Source: CAD feature listing. Evaluate the final solid. Frame: model axes, mm. Coordinates: 2 decimals unless noted, no trailing zeros. Loops run counter-clockwise (first coordinate to the right, second up) from the corner with the lowest first, then second, coordinate; pieces in that order, holes last. Notation, with made-up numbers: M 17.25,22 L 57.25,22 A28 ccw 57.25,52 Z; hole C 47,57.25 d11. An arc over 180 degrees is marked long. One line per question, with ' | ' between items. Start each with the question number.
1. Mould query, pull axis Z, two halves, no side actions, for faces 1 (the flat face through (-11.5, 1, -10)), 2 (the cylindrical face through (-1.39, 1.48, -16.01)), 3 (the flat face through (-6, 1, 0)), 4 (the cylindrical face through (-1.3, 1.5, -4.1)). Classes: pulls with the +Z half, pulls with the -Z half, needs draft (parallel to the pull), parting line crosses it, or undercut.
2. Section query C-C, the plane y = 1.65. Output: boundary loops of the cut face in (x, z).
3. Ray query, probe 1 along Z at (x, y) = (-9, 1.5); probe 2 along X at (y, z) = (1.4, -6.25); probe 3 along Z at (x, y) = (-1.25, 0.85). Return the intervals inside material, ascending.
4. Section query B-B, the plane x = -9. Output: boundary loops of the cut face in (y, z), and give its area (3 significant figures).
5. Section query A-A, the plane z = -5. Output: boundary loops of the cut face in (x, y), and give its area (3 significant figures).
Autodesk Inventor part; units mm, degrees
ref_plane "YZ Plane" through (0, 0, 0) normal (1, 0, 0) x (0, 1, 0)
ref_plane "XZ Plane" through (0, 0, 0) normal (0, 1, 0) x (-1, 0, 0)
ref_plane "XY Plane" through (0, 0, 0) normal (0, 0, 1) x (1, 0, 0)
sketch "Esquisse1" plane through (0, 0, 0) normal (0, 1, 0) x (-1, 0, 0)
  line L0 (0, 0) -> (11.5, 0)
  line L1 (11.5, 0) -> (11.5, -20)
  line L2 (11.5, -20) -> (0, -20)
  line L3 (0, -20) -> (0, 0)
  line L4 (9, 0) -> (9, -20) construction
  line L5 (5.75, 0) -> (5.75, -20) construction
  line L6 (11.5, -10) -> (0, -10) construction
  circle A0 centre (9, -15) radius 1.5
  circle A1 centre (9, -5) radius 1.5
  circle A2 centre (2.5, -15) radius 1.5
  circle A3 centre (2.5, -5) radius 1.5
  dimension "d0" = 20
  dimension "d1" = 11.5
  dimension "d2" = 3
  dimension "d3" = 2.5
  dimension "d4" = 10
extrude "Extrusion1" add sketch "Esquisse1" along normal blind 3
sketch "Esquisse2" plane through (0, 0, 0) normal (0, -1, 0) x (1, 0, 0)
  circle A0 centre (-2.5, -5) radius 1.5
  circle A1 centre (-2.5, -15) radius 1.5
  circle A2 centre (-9, -5) radius 1.5
  circle A3 centre (-9, -15) radius 1.5
  line L0 (0, 0) -> (-11.5, 0)
  line L1 (-11.5, 0) -> (-11.5, -20)
  line L2 (-11.5, -20) -> (0, -20)
  line L3 (0, -20) -> (0, 0)
  line L4 (-11.5, 0) -> (-12, 0)
  line L5 (-12, 0) -> (-12, -20)
  line L6 (-12, -20) -> (-11.5, -20)
  line L7 (-11.5, -20) -> (-11.5, 0)
  dimension "d7" = 0.5
extrude "Extrusion2" [suppressed]
properties part number "adapter_bottom"
Taken from the geometry:
1) face 1: needs draft | face 2: undercut | face 3: pulls with the +Z half | face 4: undercut
2) outline: M -11.5,-20 L 0,-20 L 0,0 L -11.5,0 Z; hole C -9,-15 d3; hole C -9,-5 d3; hole C -2.5,-15 d3; hole C -2.5,-5 d3
3) probe 1: -20 to -16.5, -13.5 to -6.5, -3.5 to 0 | probe 2: -11.5 to -9.83, -8.17 to -3.33, -1.67 to 0 | probe 3: -20 to -15.83, -14.17 to -5.83, -4.17 to 0
4) outline: M 0,-20 L 3,-20 L 3,-16.5 L 0,-16.5 Z; M 0,-13.5 L 3,-13.5 L 3,-6.5 L 0,-6.5 Z; M 0,-3.5 L 3,-3.5 L 3,0 L 0,0 Z | area: 42.0 mm^2
5) outline: M -11.5,0 L -10.5,0 L -10.5,3 L -11.5,3 Z; M -7.5,0 L -4,0 L -4,3 L -7.5,3 Z; M -1,0 L 0,0 L 0,3 L -1,3 Z | area: 16.5 mm^2
